```python
from build123d import *

# Parameters (mm, degrees)
F0_W     = 140
F0_H     = 120
F0_R     = 1.6002
F1_DEPTH = 32.5
F2_W     = 52
F2_H     = 26.5
F3_DEPTH = 120
F4_W     = 114
F4_H     = 29.5
F5_DEPTH = 100


with BuildPart() as f1:
    # F0 (on Top) → F1 (new body)
    with BuildSketch(Plane.XY):
        Rectangle(F0_W, F0_H)
        Circle(F0_R, mode=Mode.SUBTRACT)
        with BuildLine():
            Line((70, 60), (70, -60))
            ThreePointArc((70, -60), (100, 0), (70, 60))
        make_face()
    extrude(amount=F1_DEPTH)

    # F2 (on face) → F3 (cut)
    with BuildSketch(Plane(origin=(0, 60, 0), x_dir=(-1, 0, 0), z_dir=(0, 1, 0))):
        with Locations((-41, 16.25)):
            Rectangle(F2_W, F2_H)
    extrude(amount=-F3_DEPTH, mode=Mode.SUBTRACT)

    # F4 (on face) → F5 (cut)
    with BuildSketch(Plane(origin=(-70, 0, 0), x_dir=(0, -1, 0), z_dir=(-1, 0, 0))):
        with Locations((0, 14.75)):
            Rectangle(F4_W, F4_H)
    extrude(amount=-F5_DEPTH, mode=Mode.SUBTRACT)


solid = f1.part
```
Geometry check sheet. Reference: the model listing, model coordinates, mm. A direction names the side the tool comes from. Round coordinates to 2 decimals unless told otherwise and drop trailing zeros. Write each loop counter-clockwise with the first axis right and the second up, starting at its lowest first coordinate (ties: lowest second). Pieces come first, ordered by that corner, then holes. Notation, with made-up numbers: (-19.5, 84.25) -> (6.5, 84.25) arc R36 ccw to (6.5, 122.25) -> close; hole circle Ø8 at (-8.5, 60.5). An arc over 180 degrees is marked (long way). Put each result on its own line as item: value.
1) Access from +Z, -Z, +X, -X, +Y, -Y to the whole of each face (thin tool, end or side, straight path). Record for faces 4 (the face through (-21, -57, 15)), 5 (the face through (99.994, -0.974, 16.022)).
Recorded:
face 4: -Z, -X
face 5: +Z, -Z, +X
2) Cross-section at D-D, the plane y = 16.5. Enter the section's corners in (x, z), plus the area to 3 significant figures.
Recorded:
outline: (-70, 29.5) -> (67, 29.5) -> (67, 3) -> (30, 3) -> (30, 0) -> (98.16, 0) -> (98.16, 32.5) -> (-70, 32.5) -> close
area: 1,530 mm2
3) Release check for a two-part mould opening along Z. For faces 1 (the face through (47, 1, 3)), 2 (the face through (52, 1, 0)), 3 (the face through (-1.27, -0.974, 30.979)) record: pulls with the +Z half, pulls with the -Z half, needs draft (parallel to the pull), parting line crosses it, or undercut.
Recorded:
face 1: undercut
face 2: pulls with the -Z half
face 3: needs draft
4) Thickness scan on probe 1 along Y at (x, z) = (0, 30.85); probe 2 along Y at (x, z) = (-26, 13); probe 3 along Z at (x, y) = (11, 52). Record the ranges inside material, lowest first. Write a range as from..to.
Recorded:
probe 1: y = -60..-1.6, 1.6..60
probe 2: y = -60..-57, 57..60
probe 3: z = 29.5..32.5
5) Cross-section at A-A, the plane z = 22. Enter the section's corners in (x, y).
Recorded:
outline: (-70, -60) -> (15, -60) -> (15, -57) -> (-70, -57) -> close; (-70, 57) -> (15, 57) -> (15, 60) -> (-70, 60) -> close; (67, -60) -> (70, -60) arc R75 ccw to (70, 60) -> (67, 60) -> close
6) Cross-section at C-C, the plane x = -30.5. Enter the section's corners in (y, z), plus the area to 3 significant figures.
Recorded:
outline: (-60, 0) -> (-57, 0) -> (-57, 29.5) -> (57, 29.5) -> (57, 0) -> (60, 0) -> (60, 32.5) -> (-60, 32.5) -> close
area: 537 mm2
7) Cross-section at B-B, the plane x = 41.5. Enter the section's corners in (y, z), plus the area to 3 significant figures.
Recorded:
outline: (-60, 0) -> (60, 0) -> (60, 3) -> (-60, 3) -> close; (-60, 29.5) -> (60, 29.5) -> (60, 32.5) -> (-60, 32.5) -> close
area: 720 mm2
8) Depth check by flat-ended pin: P1, Ø5, axis at y = 35.5, z = 8, coming from the +X side; P2, Ø1.5, axis at y = -58, z = 22.5, coming from the +X side; P3, Ø1, axis at x = 80.5, y = -46, coming from the -Z side; P4, Ø8, axis at y = -15.5, z = 19.5, coming from the -X side. Enter the tip coordinate at first touch or a pass-through.
Recorded:
P1: stops at x = 92.35
P2: stops at x = 73.45
P3: stops at z = 0
P4: stops at x = 67
